from build123d import *

# Parameters (mm, degrees)
BOSS_EXTRUDE1_DEPTH      = 54
BOSS_EXTRUDE1_DEPTH_BACK = 1
SKETCH1_R                = 52.838
CUT_EXTRUDE1_DEPTH       = 53


with BuildPart() as part:
    # Sketch1 → Boss-Extrude1 (new, two sides: drawn at the far end of the back side and taken through both)
    with BuildSketch(Plane(origin=(0, 0, 0), x_dir=(1, 0, 0), z_dir=(0, 1, 0)).offset(-BOSS_EXTRUDE1_DEPTH_BACK)):
        with BuildLine():
            Line((-51.240048916, 38.94945257), (-51.240048916, 13.94945257))
            ThreePointArc((-51.240048916, 13.94945257), (9.321392976, -35.38854743), (69.882834868, 13.94945257))
            Line((69.882834868, 13.94945257), (69.882834868, 38.94945257))
            ThreePointArc((69.882834868, 38.94945257), (9.321392976, 88.28745257), (-51.240048916, 38.94945257))
        make_face()
        with Locations(Location((9.321392976, 26.44945257, 0), (0, 0, 270))):
            Circle(SKETCH1_R, mode=Mode.SUBTRACT)
    extrude(amount=BOSS_EXTRUDE1_DEPTH + BOSS_EXTRUDE1_DEPTH_BACK)

    # Sketch2 → Cut-Extrude1 (cut)
    with BuildSketch(Plane.XY):
        with BuildLine():
            Line((-3.360607024, 20.5), (-3.360607024, -1))
            Line((-3.360607024, -1), (22.003392976, -1))
            Line((22.003392976, -1), (22.003392976, 20.5))
            ThreePointArc((22.003392976, 20.5), (9.321392976, 33.182), (-3.360607024, 20.5))
        make_face()
    extrude(amount=CUT_EXTRUDE1_DEPTH, mode=Mode.SUBTRACT)


solid = part.part
CAD build for the part. Positions are in the model's coordinates, mm. A direction names the side the tool comes from. Round coordinates to 2 decimals unless told otherwise and drop trailing zeros. Loops run counter-clockwise (first coordinate to the right, second up) from the corner with the lowest first, then second, coordinate; pieces in that order, holes last. Notation, with made-up numbers: (1, 19.25) - (50, 19.25) arc R21 cw to (50, 37.25) - close; hole circle Ø2 at (45.5, 25). An arc over 180 degrees is marked (long way). Put each result on its own line as item: value.
1. Slice it at C-C on y = 18. List the corners of the cut face in (x, z), and give its area (3 significant figures).
Geometry check:
outline: (-51.24, -38.95) arc R61.84 ccw to (69.88, -38.95) - (69.88, -13.95) arc R61.84 ccw to (22, 34.07) - (22, 24.84) arc R52.84 cw (long way) to (-3.36, 24.84) - (-3.36, 34.07) arc R61.84 ccw to (-51.24, -13.95) - close
area: 2,970 mm²
2. Pin check, flat tips, straight feed: P1, Ø2, axis at x = 17, y = 42.5, coming from the -Z side; P2, Ø10, axis at x = 57.5, y = 28, coming from the +Z side; P3, Ø4, axis at y = 42, z = -72, coming from the +X side. Stop position of each tip, or through.
Geometry check:
P1: z = -87.93
P2: z = 17.82
P3: x = 53.22
3. Slice it at A-A on z = -1. List the corners of the cut face in (x, y).
Geometry check:
outline: (-47.04, -1) - (-36.98, -1) - (-36.98, 54) - (-47.04, 54) - close; (55.63, -1) - (65.68, -1) - (65.68, 54) - (55.63, 54) - close
4. Slice it at B-B on x = 32.5. List the corners of the cut face in (y, z).
Geometry check:
outline: (-1, -83.78) - (54, -83.78) - (54, -73.93) - (-1, -73.93) - close; (-1, 21.03) - (54, 21.03) - (54, 30.88) - (-1, 30.88) - close
5. Slice it at D-D on y = 42.5. List the corners of the cut face in (x, z), and give its area (3 significant figures).
Geometry check:
outline: (-51.24, -38.95) arc R61.84 ccw to (69.88, -38.95) - (69.88, -13.95) arc R61.84 ccw to (-51.24, -13.95) - close; hole circle Ø105.68 at (9.32, -26.45)
area: 3,200 mm²
6. 3-axis set-ups, long thin cutter, end or side, ignore diameter. For faces 1 (the cylindrical face through (10.505, 26.115, -88.276)), 2 (the flat face through (22.003, 10, 29)): which of +Z, -Z, +X, -X, +Y, -Y reach the whole face in a straight line?
Geometry check:
face 1: -Z, +Y, -Y
face 2: +Z, -Y
7. Wall check: line 1 (Z direction, x = -23, y = 41); line 2 (X direction, y = 8.5, z = 12.5); line 3 (Z direction, x = 18, y = 31.5). Give the ranges that are in metal, low to high.
Geometry check:
line 1: -79.17 to -68.25, 15.35 to 26.27
line 2: -38.71 to -26.38, 45.03 to 57.35
line 3: -87.68 to -78.57, 25.67 to 34.78
8. Two-plate mould, pull along X, no slides. Class faces 3 (the cylindrical face through (9.6, 33.18, 30.05)), 4 (the flat face through (-51.24, 26, -27)), 5 (the flat face through (-18, -1, -73)): released by +X, released by -X, zero draft, split by the parting line, or undercut.
Geometry check:
face 3: undercut
face 4: released by -X
face 5: zero draft
